Read the model definition and answer for the solid it produces. Units are mm, in the model's axes. A direction names the side the tool comes from. Give positions to 0.01 mm unless a question says otherwise; leave off trailing zeros. Write each loop counter-clockwise with the first axis right and the second up, starting at its lowest first coordinate (ties: lowest second). Pieces come first, ordered by that corner, then holes. Notation, with made-up numbers: (49, 68.25) - (76, 68.25) arc R23 cw to (76, 93.25) - close; hole circle Ø1 at (40.5, 43.25). An arc over 180 degrees is marked (long way). Use CSV: the item, a comma, the result in double quotes. Start each with the question number.
from build123d import *

# Parameters (mm, degrees)
F0_W     = 80
F0_H     = 40
F1_DEPTH = 6
F2_R     = 3.5
F3_DEPTH = 25
F5_DEPTH = 25
F6_W     = 20.5047205091
F6_H     = 1.8820744008
F6_W_2   = 18.622642383
F6_H_2   = 2.0801890641
F6_W_3   = 19.7122655809
F6_H_3   = 2.2783023305
F7_DEPTH = 25


with BuildPart() as f1:
    # F0 (on Right) → F1 (new body)
    with BuildSketch(Plane.YZ):
        with Locations((-26.8443413079, 17.3577393824)):
            Rectangle(F0_W, F0_H)
    extrude(amount=F1_DEPTH)

    # F2 (on face) → F3 (cut)
    with BuildSketch(Plane.YZ.offset(6)):
        with Locations((-52.0895607769, 14.3577393824)):
            Circle(F2_R)
    extrude(amount=-F3_DEPTH, mode=Mode.SUBTRACT)

    # F4 (on face) → F5 (cut)
    with BuildSketch(Plane.YZ.offset(6)):
        with BuildLine():
            ThreePointArc((-3.5001474581, 5.8439973669), (-3.4839255473, 6.137753605), (-3.478515805, 6.4319076676))
            ThreePointArc((-3.478515805, 6.4319076676), (-3.8394647971, 8.807807434), (-4.8897407299, 10.9693125439))
            ThreePointArc((-4.8897407299, 10.9693125439), (-7.8217234118, 13.5472340406), (-11.6246055812, 14.4305736675))
            ThreePointArc((-11.6246055812, 14.4305736675), (-15.2948749769, 13.4629390764), (-18.1060345681, 10.9125320711))
            ThreePointArc((-18.1060345681, 10.9125320711), (-19.2350505337, 8.3905217189), (-19.4387102983, 5.6348483044))
            Line((-19.4387102983, 5.6348483044), (-18.8812702578, 3.3988849985))
            Line((-18.8812702578, 3.3988849985), (-4.0757613522, 3.3988849985))
            Line((-4.0757613522, 3.3988849985), (-3.5001474581, 5.8439973669))
        make_face()
        with BuildLine():
            ThreePointArc((-18.8812702578, 3.3988849985), (-11.478515805, -1.5680923324), (-4.0757613522, 3.3988849985))
            Line((-4.0757613522, 3.3988849985), (-18.8812702578, 3.3988849985))
        make_face()
        with BuildLine():
            ThreePointArc((-19.4387102983, 5.6348483044), (-19.2350505337, 8.3905217189), (-18.1060345681, 10.9125320711))
            Line((-18.1060345681, 10.9125320711), (-21.6475948691, 24.4305736675))
            Line((-21.6475948691, 24.4305736675), (-24.1246055812, 24.4305736675))
            Line((-24.1246055812, 24.4305736675), (-19.4387102983, 5.6348483044))
        make_face()
        with BuildLine():
            ThreePointArc((-4.8897407299, 10.9693125439), (-3.8394647971, 8.807807434), (-3.478515805, 6.4319076676))
            ThreePointArc((-3.478515805, 6.4319076676), (-3.4839255473, 6.137753605), (-3.5001474581, 5.8439973669))
            Line((-3.5001474581, 5.8439973669), (0.8753944188, 24.4305736675))
            Line((0.8753944188, 24.4305736675), (-1.1863555992, 24.4305736675))
            Line((-1.1863555992, 24.4305736675), (-4.8897407299, 10.9693125439))
        make_face()
    extrude(amount=-F5_DEPTH, mode=Mode.SUBTRACT)

    # F6 (on face) → F7 (cut)
    with BuildSketch(Plane.YZ.offset(6)):
        with Locations((-50.2029955387, 22.2922516987)):
            Rectangle(F6_W, F6_H)
        with Locations((-35.6912026182, 15.4573461041)):
            Rectangle(F6_W_2, F6_H_2)
        with Locations((-49.8067680746, 7.6318744104)):
            Rectangle(F6_W_3, F6_H_3)
    extrude(amount=-F7_DEPTH, mode=Mode.SUBTRACT)


solid = f1.part
(1) Which of the six approach directions +Z, -Z, +X, -X, +Y, -Y give full straight-line access (tool end or side, diameter ignored) to faces 1 (the face through (3, -66.844, 17)), 2 (the face through (3, -50, 6.493))?
(2) For a pull along Z with two mould halves and no side action, classify faces 3 (the face through (3, -39.951, 8)), 4 (the face through (3, -27, 37.358)), 5 (the face through (6, -27, 18)) as pulls with the +Z half, pulls with the -Z half, needs draft (parallel to the pull), parting line crosses it, or undercut.
(3) The part is cut by section A-A on y = -52.5. Write down the section's boundary in (x, z), plus the area to 3 significant figures.
(4) The part is cut by section D-D on y = -23. Write down the section's boundary in (x, z), plus the area to 3 significant figures.
(5) The part is cut by section C-C on z = 20. Write down the section's boundary in (x, y), plus the area to 3 significant figures.
(6) The part is cut by section B-B on x = 3.5. Write down the section's boundary in (y, z), plus the area to 3 significant figures.
(7) Consider probe 1 along Z at (x, y) = (4.5, -41); probe 2 along Z at (x, y) = (4.25, -49); probe 3 along Z at (x, y) = (3.25, -33). Determine where each line is inside the solid, lowest interval first.
Reported:
1,face 1,"+Z, -Z, +X, -X, -Y"
1,face 2,"+X, -X"
2,face 3,"undercut"
2,face 4,"pulls with the +Z half"
2,face 5,"needs draft"
3,outline,"(0, -2.64) - (6, -2.64) - (6, 6.49) - (0, 6.49) - close; (0, 8.77) - (6, 8.77) - (6, 10.88) - (0, 10.88) - close; (0, 17.83) - (6, 17.83) - (6, 21.35) - (0, 21.35) - close; (0, 23.23) - (6, 23.23) - (6, 37.36) - (0, 37.36) - close"
3,area,"173 mm²"
4,outline,"(0, -2.64) - (6, -2.64) - (6, 19.92) - (0, 19.92) - close; (0, 24.43) - (6, 24.43) - (6, 37.36) - (0, 37.36) - close"
4,area,"213 mm²"
5,outline,"(0, -66.84) - (6, -66.84) - (6, -23.02) - (0, -23.02) - close; (0, -20.49) - (6, -20.49) - (6, -2.41) - (0, -2.41) - close; (0, -0.17) - (6, -0.17) - (6, 13.16) - (0, 13.16) - close"
5,area,"451 mm²"
6,outline,"(-66.84, -2.64) - (13.16, -2.64) - (13.16, 37.36) - (-66.84, 37.36) - close; hole (-60.46, 21.35) - (-39.95, 21.35) - (-39.95, 23.23) - (-60.46, 23.23) - close; hole (-59.66, 6.49) - (-39.95, 6.49) - (-39.95, 8.77) - (-59.66, 8.77) - close; hole circle Ø7 at (-52.09, 14.36); hole (-45, 14.42) - (-26.38, 14.42) - (-26.38, 16.5) - (-45, 16.5) - close; hole (-24.12, 24.43) - (-18.88, 3.4) arc R8 ccw to (-4.08, 3.4) - (0.88, 24.43) - (-1.19, 24.43) - (-4.89, 10.97) arc R8 ccw to (-18.11, 10.91) - (-21.65, 24.43) - close"
6,area,"2,760 mm²"
7,probe 1,"-2.64 to 6.49, 8.77 to 14.42, 16.5 to 21.35, 23.23 to 37.36"
7,probe 2,"-2.64 to 6.49, 8.77 to 12.71, 16 to 21.35, 23.23 to 37.36"
7,probe 3,"-2.64 to 14.42, 16.5 to 37.36"
